The model under review builds one solid part; all positions refer to its coordinate system, in mm. Face numbers are marked on the shaded views. A direction names the side the tool comes from. Round coordinates to 2 decimals unless told otherwise and drop trailing zeros. Loops run counter-clockwise (first coordinate to the right, second up) from the corner with the lowest first, then second, coordinate; pieces in that order, holes last. Notation, with made-up numbers: (35.5, 85.25) -> (66.5, 85.25) arc R17 cw to (66.5, 103.25) -> close; hole circle Ø7 at (55.5, -35). An arc over 180 degrees is marked (long way). Use a Markdown table: item, result. Add a question column.
1) Insertion check: pin 1 (8 mm diameter, centred on x = -2.5, y = 2.5, fed in from -Z); pin 2 (5 mm diameter, centred on y = 7, z = 10, fed in from +X); pin 3 (3.5 mm diameter, centred on y = 0, z = 7.5, fed in from -X); pin 4 (3 mm diameter, centred on x = 6, z = -0.5, fed in from +Y). Each pin has a flat end and moves straight along its axis. Give the tip position at first contact, or say it passes through.
2) Consider section A-A on z = 4.5. Give the boundary of the cut face in (x, y).
3) Consider section D-D on x = -11.5. Give the boundary of the cut face in (y, z), plus the area to 3 significant figures.
4) Consider section B-B on y = 5.75. Give the boundary of the cut face in (x, z).
5) Wall thickness on probe 1 along Z at (x, y) = (7, 6); probe 2 along Y at (x, z) = (0, 0.45); probe 3 along X at (y, z) = (-12.75, 8): over which ranges is each line inside the solid? List them lowest first.
6) For the marked faces 1, 2, 3 and 4, list the 3-axis set-ups (+Z, -Z, +X, -X, +Y, -Y) from which the entire face can be reached by the end or side of a thin tool; tool diameter is ignored.
7) Mouldability with a two-part tool opening along X and no side actions: class the marked faces 5, 6 and 7 as released by +X, released by -X, zero draft, split by the parting line, or undercut.
8) Consider section C-C on z = 7.5. Give the boundary of the cut face in (x, y), plus the area to 3 significant figures.
from build123d import *

# Parameters (mm, degrees)
SKETCH1_W           = 47
SKETCH1_H           = 27
BOSS_EXTRUDE1_DEPTH = 15
SKETCH2_W           = 45
SKETCH2_H           = 13
CUT_EXTRUDE1_DEPTH  = 27
SKETCH3_W           = 55
SKETCH3_H           = 23
SKETCH3_W_2         = 45
SKETCH3_H_2         = 13
BOSS_EXTRUDE2_DEPTH = 1
SKETCH4_R           = 1.5
CUT_EXTRUDE2_DEPTH  = 17
SKETCH5_R           = 1.5
CUT_EXTRUDE3_DEPTH  = 47


with BuildPart() as part:
    # Sketch1 → Boss-Extrude1 (new body)
    with BuildSketch(Plane.XY):
        Rectangle(SKETCH1_W, SKETCH1_H)
    extrude(amount=BOSS_EXTRUDE1_DEPTH)

    # Sketch2 → Cut-Extrude1 (cut)
    with BuildSketch(Plane(origin=(0, 13.5, 0), x_dir=(1, 0, 0), z_dir=(0, 1, 0))):
        with Locations((0, -7.5)):
            Rectangle(SKETCH2_W, SKETCH2_H)
    extrude(amount=-CUT_EXTRUDE1_DEPTH, mode=Mode.SUBTRACT)

    # Sketch3 → Boss-Extrude2 (add)
    with BuildSketch(Plane.XZ.offset(13.5)):
        with Locations((0, 7.5)):
            Rectangle(SKETCH3_W, SKETCH3_H)
        with Locations((0, 7.5)):
            Rectangle(SKETCH3_W_2, SKETCH3_H_2, mode=Mode.SUBTRACT)
    extrude(amount=BOSS_EXTRUDE2_DEPTH)

    # Sketch4 → Cut-Extrude2 (cut)
    with BuildSketch(Plane.XY.offset(15)):
        Circle(SKETCH4_R)
    extrude(amount=-CUT_EXTRUDE2_DEPTH, mode=Mode.SUBTRACT)

    # Sketch5 → Cut-Extrude3 (cut)
    with BuildSketch(Plane.ZY.offset(23.5)):
        with Locations(Location((7.5, 0, 0), (0, 0, 270))):
            Circle(SKETCH5_R)
    extrude(amount=-CUT_EXTRUDE3_DEPTH, mode=Mode.SUBTRACT)


solid = part.part
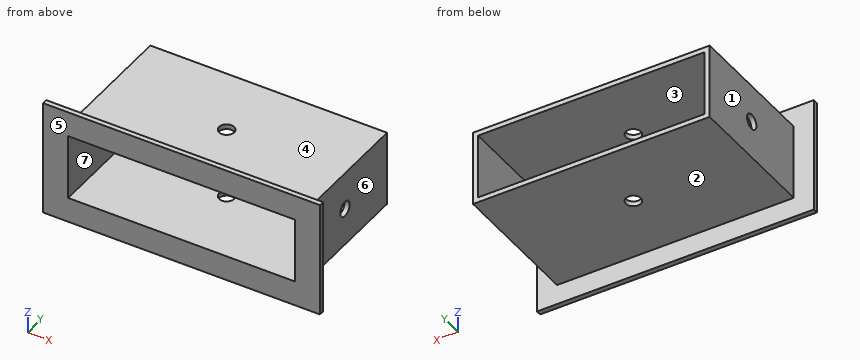
Result set:
| question | item | result |
|---|---|---|
| 1 | pin 1 | z = 0 |
| 1 | pin 2 | x = 23.5 |
| 1 | pin 3 | x = -23.5 |
| 1 | pin 4 | y = 13.5 |
| 2 | outline | (-27.5, -14.5) -> (-22.5, -14.5) -> (-22.5, 13.5) -> (-23.5, 13.5) -> (-23.5, -13.5) -> (-27.5, -13.5) -> close; (22.5, -14.5) -> (27.5, -14.5) -> (27.5, -13.5) -> (23.5, -13.5) -> (23.5, 13.5) -> (22.5, 13.5) -> close |
| 3 | outline | (-14.5, -4) -> (-13.5, -4) -> (-13.5, 0) -> (13.5, 0) -> (13.5, 1) -> (-14.5, 1) -> close; (-14.5, 14) -> (13.5, 14) -> (13.5, 15) -> (-13.5, 15) -> (-13.5, 19) -> (-14.5, 19) -> close |
| 3 | area | 64.0 mm2 |
| 4 | outline | (-23.5, 0) -> (23.5, 0) -> (23.5, 15) -> (-23.5, 15) -> close; hole (-22.5, 1) -> (22.5, 1) -> (22.5, 14) -> (-22.5, 14) -> close |
| 5 | probe 1 | 0 to 1, 14 to 15 |
| 5 | probe 2 | -14.5 to -1.5, 1.5 to 13.5 |
| 5 | probe 3 | -23.5 to -22.5, 22.5 to 23.5 |
| 6 | face 1 | +Z, -Z, -X, +Y |
| 6 | face 2 | -Z, +X, -X, +Y |
| 6 | face 3 | +Y, -Y |
| 6 | face 4 | +Z, +X, -X, +Y |
| 7 | face 5 | zero draft |
| 7 | face 6 | released by +X |
| 7 | face 7 | undercut |
| 8 | outline | (-27.5, -14.5) -> (-22.5, -14.5) -> (-22.5, -1.5) -> (-23.5, -1.5) -> (-23.5, -13.5) -> (-27.5, -13.5) -> close; (-23.5, 1.5) -> (-22.5, 1.5) -> (-22.5, 13.5) -> (-23.5, 13.5) -> close; (22.5, -14.5) -> (27.5, -14.5) -> (27.5, -13.5) -> (23.5, -13.5) -> (23.5, -1.5) -> (22.5, -1.5) -> close; (22.5, 1.5) -> (23.5, 1.5) -> (23.5, 13.5) -> (22.5, 13.5) -> close |
| 8 | area | 58.0 mm2 |
